```python
from build123d import *

# Parameters (mm, degrees)
F0_W     = 18
F0_H     = 11
F1_DEPTH = 18
F2_R     = 5


with BuildPart() as f1:
    # F0 (on Top) → F1 (new body)
    with BuildSketch(Plane.XY):
        with Locations((-0.382075, 22.777358)):
            Rectangle(F0_W, F0_H)
        with BuildLine():
            Line((-9.382075, 10.277358), (-9.382075, 9.877358))
            Line((-9.382075, 9.877358), (-8.383446, 9.929694))
            Line((-8.383446, 9.929694), (-5.037793, 13.645418))
            Line((-5.037793, 13.645418), (-4.852757, 10.11473))
            Line((-4.852757, 10.11473), (-3.390298, 10.191374))
            Line((-3.390298, 10.191374), (-0.044645, 13.907098))
            Line((-0.044645, 13.907098), (0.14039, 10.37641))
            Line((0.14039, 10.37641), (1.602849, 10.453054))
            Line((1.602849, 10.453054), (4.968313, 14.190779))
            Line((4.968313, 14.190779), (5.091545, 11.839359))
            Line((5.091545, 11.839359), (8.617925, 12.024169))
            Line((8.617925, 12.024169), (8.617925, 10.820698))
            Line((8.617925, 10.820698), (8.617925, 10.277358))
            Line((8.617925, 10.277358), (18.368002, 10.277358))
            ThreePointArc((18.368002, 10.277358), (20.368002, 12.277358), (22.368002, 10.277358))
            ThreePointArc((22.368002, 10.277358), (21.190878, 8.454483), (19.045127, 8.777358))
            Line((19.045127, 8.777358), (8.617925, 8.777358))
            Line((8.617925, 8.777358), (8.617925, -6.222642))
            Line((8.617925, -6.222642), (19.045127, -6.222642))
            ThreePointArc((19.045127, -6.222642), (21.190878, -5.899766), (22.368002, -7.722642))
            ThreePointArc((22.368002, -7.722642), (20.368002, -9.722642), (18.368002, -7.722642))
            Line((18.368002, -7.722642), (8.617925, -7.722642))
            Line((8.617925, -7.722642), (8.617925, -8.364536))
            Line((8.617925, -8.364536), (5.153458, -8.364536))
            Line((5.153458, -8.364536), (5.153458, -11.258175))
            Line((5.153458, -11.258175), (1.617925, -7.722642))
            Line((1.617925, -7.722642), (0.153458, -7.722642))
            Line((0.153458, -7.722642), (0.153458, -11.658175))
            Line((0.153458, -11.658175), (-3.782075, -7.722642))
            Line((-3.782075, -7.722642), (-4.846542, -7.722642))
            Line((-4.846542, -7.722642), (-4.846542, -11.258175))
            Line((-4.846542, -11.258175), (-8.382075, -7.722642))
            Line((-8.382075, -7.722642), (-9.382075, -7.722642))
            Line((-9.382075, -7.722642), (-9.382075, -14.722642))
            Line((-9.382075, -14.722642), (25.617925, -14.722642))
            Line((25.617925, -14.722642), (25.617925, 17.277358))
            Line((25.617925, 17.277358), (8.617925, 17.277358))
            Line((8.617925, 17.277358), (-9.382075, 17.277358))
            Line((-9.382075, 17.277358), (-9.382075, 10.277358))
        make_face()
        Polygon((-10.490221, 31.022026), (-9.382075, 9.877358), (-9.382075, 10.277358), (-9.382075, 17.277358), (-9.382075, 28.277358), (8.617925, 28.277358), (8.617925, 32.023441), align=None)
    extrude(amount=F1_DEPTH)

    # F2
    f2_edges = [f1.edges().sort_by_distance(p)[0] for p in [
        (8.617925, 17.277358, 9),
        (25.617925, 17.277358, 9),
        (25.617925, -14.722642, 9),
    ]]
    fillet(f2_edges, radius=F2_R)


solid = f1.part
```
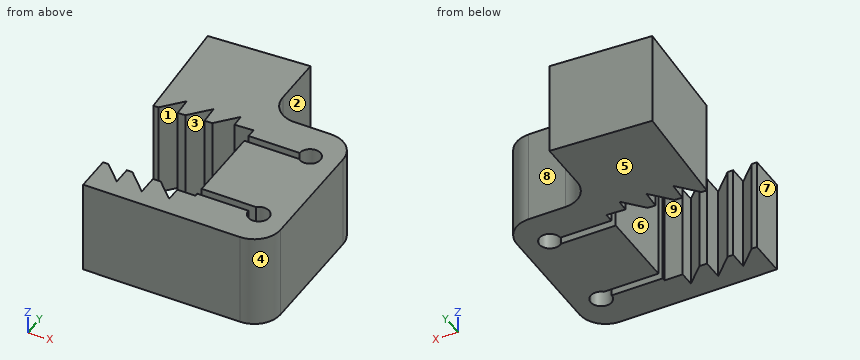
Verification items for the finished model (mm, model axes). Face numbers are marked on the shaded views. A direction names the side the tool comes from. Round coordinates to 2 decimals unless told otherwise and drop trailing zeros. Loops run counter-clockwise (first coordinate to the right, second up) from the corner with the lowest first, then second, coordinate; pieces in that order, holes last. Notation, with made-up numbers: (-6, -10) -> (10, -10) arc R18 ccw to (10, -4) -> close; hole circle Ø3 at (49.25, 7.5). An arc over 180 degrees is marked (long way). Answer as a JSON object with one key per item and string values.
Q1. Section check A-A (x = 17.5). Record the boundary of the cut face in (y, z).
Data:
{"outline": "(-14.72, 0) -> (-7.72, 0) -> (-7.72, 18) -> (-14.72, 18) -> close; (-6.22, 0) -> (8.78, 0) -> (8.78, 18) -> (-6.22, 18) -> close; (10.28, 0) -> (17.28, 0) -> (17.28, 18) -> (10.28, 18) -> close"}
Q2. Section check D-D (x = -6). Record the boundary of the cut face in (y, z).
Data:
{"outline": "(-14.72, 0) -> (-10.1, 0) -> (-10.1, 18) -> (-14.72, 18) -> close; (12.58, 0) -> (31.26, 0) -> (31.26, 18) -> (12.58, 18) -> close"}
Q3. Section check C-C (y = 3.5). Record the boundary of the cut face in (x, z), then the cut area to 3 significant figures.
Data:
{"outline": "(8.62, 0) -> (25.62, 0) -> (25.62, 18) -> (8.62, 18) -> close", "area": "306 mm2"}
Q4. Section check B-B (x = 8). Record the boundary of the cut face in (y, z).
Data:
{"outline": "(-14.72, 0) -> (-8.36, 0) -> (-8.36, 18) -> (-14.72, 18) -> close; (11.99, 0) -> (31.99, 0) -> (31.99, 18) -> (11.99, 18) -> close"}
Q5. Go/stop test with flat-tipped pins: P1, Ø1, axis at y = 24, z = 9, coming from the -X side; P2, Ø1.8, axis at y = -10, z = 5.5, coming from the -X side; P3, Ø4.5, axis at y = 4, z = 12, coming from the -X side. Record where each tip stops, or that it passes through.
Data:
{"P1": "stops at x = -10.15", "P2": "stops at x = -9.38", "P3": "stops at x = 8.62"}
Q6. Scan lines: line 1 (Y direction, x = 16.5, z = 15); line 2 (Y direction, x = 9, z = 9.25); line 3 (X direction, y = 13, z = 14.5). Record each from-to range of solid material in increasing order. Write a range as from..to.
Data:
{"line 1": "y = -14.72..-7.72, -6.22..8.78, 10.28..17.28", "line 2": "y = -14.72..-7.72, -6.22..8.78, 10.28..20.36", "line 3": "x = -9.55..-5.62, -5..-0.86, 0..3.9, 5.03..25.57"}
Q7. Draft check along Y on the marked faces 1, 2, 3 and 4. Enter one of: pulls with the +Y half, pulls with the -Y half, needs draft (parallel to the pull), parting line crosses it, or undercut.
Data:
{"face 1": "undercut", "face 2": "needs draft", "face 3": "undercut", "face 4": "pulls with the -Y half"}
Q8. Access from +Z, -Z, +X, -X, +Y, -Y to the whole of each face (thin tool, end or side, straight path). Record for the marked faces 5, 6, 7, 8 and 9.
Data:
{"face 5": "-Z, +X, -X, +Y, -Y", "face 6": "+Z, -Z, -X", "face 7": "+Z, -Z, -X, -Y", "face 8": "+Z, -Z, +X, +Y", "face 9": "+Z, -Z"}
